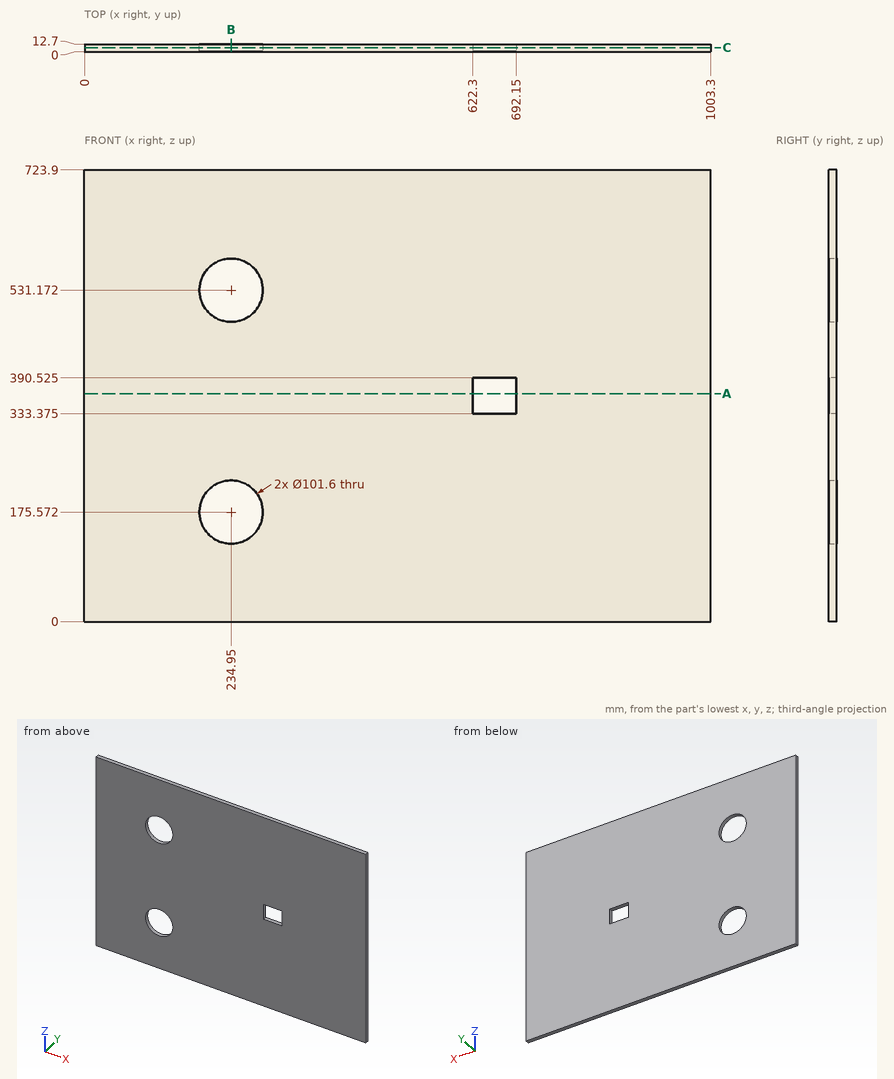
Print and shaded views of the part. All mm, measured from the part's lowest x, y and z. Round coordinates to 2 decimals unless told otherwise and drop trailing zeros. Order: outer loops, then holes, each group sorted by start corner. A loop starts at its lowest first (then second) coordinate and runs counter-clockwise, first axis right, second up.
Q1. Slice it at C-C (y = 6.75). Write the cut outline in (x, z) (3 decimals).
Q2. Slice it at A-A (z = 365.5). Write the cut outline in (x, y).
Q3. Wall check: L1, parallel to Z at x = 234.95, y = 5.25; L2, parallel to Z at x = 687, y = 9.5 (3 decimals); L3, parallel to X at y = 3.25, z = 181. Give the ranges that are in metal, low to high.
Q4. Slice it at B-B (x = 234.95). Write the cut outline in (y, z).
Results below:
1. outline: (0, 0) - (1003.3, 0) - (1003.3, 723.9) - (0, 723.9) - close; hole circle Ø101.6 at (234.95, 175.572); hole circle Ø101.6 at (234.95, 531.172); hole (622.3, 333.375) - (692.15, 333.375) - (692.15, 390.525) - (622.3, 390.525) - close
2. outline: (0, 0) - (622.3, 0) - (622.3, 12.7) - (0, 12.7) - close; (692.15, 0) - (1003.3, 0) - (1003.3, 12.7) - (692.15, 12.7) - close
3. L1: z = 0 to 124.77, 226.37 to 480.37, 581.97 to 723.9
3. L2: z = 0 to 333.375, 390.525 to 723.9
3. L3: x = 0 to 184.44, 285.46 to 1003.3
4. outline: (0, 0) - (12.7, 0) - (12.7, 124.77) - (0, 124.77) - close; (0, 226.37) - (12.7, 226.37) - (12.7, 480.37) - (0, 480.37) - close; (0, 581.97) - (12.7, 581.97) - (12.7, 723.9) - (0, 723.9) - close
